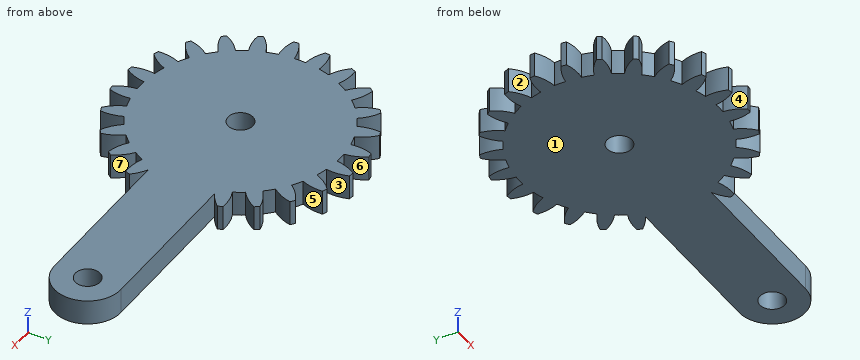
```python
from build123d import *

# Parameters (mm, degrees)
SKETCH1_R           = 1.5
BOSS_EXTRUDE1_DEPTH = 3
SCALE1_SCALE        = 1.9


with BuildPart() as part:
    # Sketch1 → Boss-Extrude1 (new body)
    with BuildSketch(Plane.XY):
        with BuildLine():
            ThreePointArc((31, -4), (35, 0), (31, 4))
            Line((31, 4), (11.967993881, 4))
            ThreePointArc((11.967993881, 4), (12.864888434, 4.573115684), (13.63194632, 5.311020574))
            ThreePointArc((13.63194632, 5.311020574), (13.516357561, 5.598658616), (13.394700346, 5.883783021))
            ThreePointArc((13.394700346, 5.883783021), (12.067442445, 5.825370588), (10.794615193, 5.444665539))
            ThreePointArc((10.794615193, 5.444665539), (10.470247132, 6.045), (10.112526268, 6.626078212))
            ThreePointArc((10.112526268, 6.626078212), (11.078640138, 7.538026423), (11.79285574, 8.658259265))
            ThreePointArc((11.79285574, 8.658259265), (11.606759368, 8.906179706), (11.415451897, 9.150101529))
            ThreePointArc((11.415451897, 9.150101529), (10.148537462, 8.750159829), (9.017614465, 8.052995056))
            ThreePointArc((9.017614465, 8.052995056), (8.548920985, 8.548920985), (8.052995056, 9.017614465))
            ThreePointArc((8.052995056, 9.017614465), (8.750159829, 10.148537462), (9.150101529, 11.415451897))
            ThreePointArc((9.150101529, 11.415451897), (8.906179706, 11.606759368), (8.658259265, 11.79285574))
            ThreePointArc((8.658259265, 11.79285574), (7.538026423, 11.078640138), (6.626078212, 10.112526268))
            ThreePointArc((6.626078212, 10.112526268), (6.045, 10.470247132), (5.444665539, 10.794615193))
            ThreePointArc((5.444665539, 10.794615193), (5.825370588, 12.067442445), (5.883783021, 13.394700346))
            ThreePointArc((5.883783021, 13.394700346), (5.598658616, 13.516357561), (5.311020574, 13.63194632))
            ThreePointArc((5.311020574, 13.63194632), (4.413811339, 12.65212943), (3.78298568, 11.482905527))
            ThreePointArc((3.78298568, 11.482905527), (3.129122255, 11.67804324), (2.465291063, 11.835980736))
            ThreePointArc((2.465291063, 11.835980736), (2.503591968, 13.163971168), (2.216494423, 14.461122103))
            ThreePointArc((2.216494423, 14.461122103), (1.909598192, 14.504838322), (1.601844607, 14.542042286))
            ThreePointArc((1.601844607, 14.542042286), (0.988802307, 13.36339701), (0.682088925, 12.070743751))
            ThreePointArc((0.682088925, 12.070743751), (0, 12.09), (-0.682088925, 12.070743751))
            ThreePointArc((-0.682088925, 12.070743751), (-0.988802307, 13.36339701), (-1.601844607, 14.542042286))
            ThreePointArc((-1.601844607, 14.542042286), (-1.909598192, 14.504838322), (-2.216494423, 14.461122103))
            ThreePointArc((-2.216494423, 14.461122103), (-2.503591968, 13.163971168), (-2.465291063, 11.835980736))
            ThreePointArc((-2.465291063, 11.835980736), (-3.129122255, 11.67804324), (-3.78298568, 11.482905527))
            ThreePointArc((-3.78298568, 11.482905527), (-4.413811339, 12.65212943), (-5.311020574, 13.63194632))
            ThreePointArc((-5.311020574, 13.63194632), (-5.598658616, 13.516357561), (-5.883783021, 13.394700346))
            ThreePointArc((-5.883783021, 13.394700346), (-5.825370588, 12.067442445), (-5.444665539, 10.794615193))
            ThreePointArc((-5.444665539, 10.794615193), (-6.045, 10.470247132), (-6.626078212, 10.112526268))
            ThreePointArc((-6.626078212, 10.112526268), (-7.538026423, 11.078640138), (-8.658259265, 11.79285574))
            ThreePointArc((-8.658259265, 11.79285574), (-8.906179706, 11.606759368), (-9.150101529, 11.415451897))
            ThreePointArc((-9.150101529, 11.415451897), (-8.750159829, 10.148537462), (-8.052995056, 9.017614465))
            ThreePointArc((-8.052995056, 9.017614465), (-8.548920985, 8.548920985), (-9.017614465, 8.052995056))
            ThreePointArc((-9.017614465, 8.052995056), (-10.148537462, 8.750159829), (-11.415451897, 9.150101529))
            ThreePointArc((-11.415451897, 9.150101529), (-11.606759368, 8.906179706), (-11.79285574, 8.658259265))
            ThreePointArc((-11.79285574, 8.658259265), (-11.078640138, 7.538026423), (-10.112526268, 6.626078212))
            ThreePointArc((-10.112526268, 6.626078212), (-10.470247132, 6.045), (-10.794615193, 5.444665539))
            ThreePointArc((-10.794615193, 5.444665539), (-12.067442445, 5.825370588), (-13.394700346, 5.883783021))
            ThreePointArc((-13.394700346, 5.883783021), (-13.516357561, 5.598658616), (-13.63194632, 5.311020574))
            ThreePointArc((-13.63194632, 5.311020574), (-12.65212943, 4.413811339), (-11.482905527, 3.78298568))
            ThreePointArc((-11.482905527, 3.78298568), (-11.67804324, 3.129122255), (-11.835980736, 2.465291063))
            ThreePointArc((-11.835980736, 2.465291063), (-13.163971168, 2.503591968), (-14.461122103, 2.216494423))
            ThreePointArc((-14.461122103, 2.216494423), (-14.504838322, 1.909598192), (-14.542042286, 1.601844607))
            ThreePointArc((-14.542042286, 1.601844607), (-13.36339701, 0.988802307), (-12.070743751, 0.682088925))
            ThreePointArc((-12.070743751, 0.682088925), (-12.09, 0), (-12.070743751, -0.682088925))
            ThreePointArc((-12.070743751, -0.682088925), (-13.36339701, -0.988802307), (-14.542042286, -1.601844607))
            ThreePointArc((-14.542042286, -1.601844607), (-14.504838322, -1.909598192), (-14.461122103, -2.216494423))
            ThreePointArc((-14.461122103, -2.216494423), (-13.163971168, -2.503591968), (-11.835980736, -2.465291063))
            ThreePointArc((-11.835980736, -2.465291063), (-11.67804324, -3.129122255), (-11.482905527, -3.78298568))
            ThreePointArc((-11.482905527, -3.78298568), (-12.65212943, -4.413811339), (-13.63194632, -5.311020574))
            ThreePointArc((-13.63194632, -5.311020574), (-13.516357561, -5.598658616), (-13.394700346, -5.883783021))
            ThreePointArc((-13.394700346, -5.883783021), (-12.067442445, -5.825370588), (-10.794615193, -5.444665539))
            ThreePointArc((-10.794615193, -5.444665539), (-10.470247132, -6.045), (-10.112526268, -6.626078212))
            ThreePointArc((-10.112526268, -6.626078212), (-11.078640138, -7.538026423), (-11.79285574, -8.658259265))
            ThreePointArc((-11.79285574, -8.658259265), (-11.606759368, -8.906179706), (-11.415451897, -9.150101529))
            ThreePointArc((-11.415451897, -9.150101529), (-10.148537462, -8.750159829), (-9.017614465, -8.052995056))
            ThreePointArc((-9.017614465, -8.052995056), (-8.548920985, -8.548920985), (-8.052995056, -9.017614465))
            ThreePointArc((-8.052995056, -9.017614465), (-8.750159829, -10.148537462), (-9.150101529, -11.415451897))
            ThreePointArc((-9.150101529, -11.415451897), (-8.906179706, -11.606759368), (-8.658259265, -11.79285574))
            ThreePointArc((-8.658259265, -11.79285574), (-7.538026423, -11.078640138), (-6.626078212, -10.112526268))
            ThreePointArc((-6.626078212, -10.112526268), (-6.045, -10.470247132), (-5.444665539, -10.794615193))
            ThreePointArc((-5.444665539, -10.794615193), (-5.825370588, -12.067442445), (-5.883783021, -13.394700346))
            ThreePointArc((-5.883783021, -13.394700346), (-5.598658616, -13.516357561), (-5.311020574, -13.63194632))
            ThreePointArc((-5.311020574, -13.63194632), (-4.413811339, -12.65212943), (-3.78298568, -11.482905527))
            ThreePointArc((-3.78298568, -11.482905527), (-3.129122255, -11.67804324), (-2.465291063, -11.835980736))
            ThreePointArc((-2.465291063, -11.835980736), (-2.503591968, -13.163971168), (-2.216494423, -14.461122103))
            ThreePointArc((-2.216494423, -14.461122103), (-1.909598192, -14.504838322), (-1.601844607, -14.542042286))
            ThreePointArc((-1.601844607, -14.542042286), (-0.988802307, -13.36339701), (-0.682088925, -12.070743751))
            ThreePointArc((-0.682088925, -12.070743751), (0, -12.09), (0.682088925, -12.070743751))
            ThreePointArc((0.682088925, -12.070743751), (0.988802307, -13.36339701), (1.601844607, -14.542042286))
            ThreePointArc((1.601844607, -14.542042286), (1.909598192, -14.504838322), (2.216494423, -14.461122103))
            ThreePointArc((2.216494423, -14.461122103), (2.503591968, -13.163971168), (2.465291063, -11.835980736))
            ThreePointArc((2.465291063, -11.835980736), (3.129122255, -11.67804324), (3.78298568, -11.482905527))
            ThreePointArc((3.78298568, -11.482905527), (4.413811339, -12.65212943), (5.311020574, -13.63194632))
            ThreePointArc((5.311020574, -13.63194632), (5.598658616, -13.516357561), (5.883783021, -13.394700346))
            ThreePointArc((5.883783021, -13.394700346), (5.825370588, -12.067442445), (5.444665539, -10.794615193))
            ThreePointArc((5.444665539, -10.794615193), (6.045, -10.470247132), (6.626078212, -10.112526268))
            ThreePointArc((6.626078212, -10.112526268), (7.538026423, -11.078640138), (8.658259265, -11.79285574))
            ThreePointArc((8.658259265, -11.79285574), (8.906179706, -11.606759368), (9.150101529, -11.415451897))
            ThreePointArc((9.150101529, -11.415451897), (8.750159829, -10.148537462), (8.052995056, -9.017614465))
            ThreePointArc((8.052995056, -9.017614465), (8.548920985, -8.548920985), (9.017614465, -8.052995056))
            ThreePointArc((9.017614465, -8.052995056), (10.148537462, -8.750159829), (11.415451897, -9.150101529))
            ThreePointArc((11.415451897, -9.150101529), (11.606759368, -8.906179706), (11.79285574, -8.658259265))
            ThreePointArc((11.79285574, -8.658259265), (11.078640138, -7.538026423), (10.112526268, -6.626078212))
            ThreePointArc((10.112526268, -6.626078212), (10.470247132, -6.045), (10.794615193, -5.444665539))
            ThreePointArc((10.794615193, -5.444665539), (12.067442445, -5.825370588), (13.394700346, -5.883783021))
            ThreePointArc((13.394700346, -5.883783021), (13.516357561, -5.598658616), (13.63194632, -5.311020574))
            ThreePointArc((13.63194632, -5.311020574), (12.864888434, -4.573115684), (11.967993881, -4))
            Line((11.967993881, -4), (31, -4))
        make_face()
        Circle(SKETCH1_R, mode=Mode.SUBTRACT)
        with Locations((31, 0)):
            Circle(SKETCH1_R, mode=Mode.SUBTRACT)
    extrude(amount=-BOSS_EXTRUDE1_DEPTH)


with BuildPart() as part_1:
    # Scale1: scaled about (5.383637445, 0, -1.5)
    add(part.part.scale(SCALE1_SCALE).moved(Location((-4.8452737, 0, 1.35))))


solid = part_1.part
```
Check sheet for the modelled part. Datum: model origin and axes. Units: mm. Face numbers are marked on the shaded views. A direction names the side the tool comes from. Round coordinates to 2 decimals unless told otherwise and drop trailing zeros. Loops run counter-clockwise (first coordinate to the right, second up) from the corner with the lowest first, then second, coordinate; pieces in that order, holes last. Notation, with made-up numbers: (84.25, 4.5) - (137.25, 4.5) arc R14 cw to (137.25, 15.5) - close; hole circle Ø9 at (51, 57). An arc over 180 degrees is marked (long way). Write item = value, one per line. Start each with the question number.
Q1. Section check C-C (z = 0.2). Count the separate pieces of the cut face and the enclosed holes in it, plus the area to 3 significant figures.
Q2. Section check D-D (x = 9). Record the boundary of the cut face in (y, z).
Q3. Release check for a two-part mould opening along Y. For the marked faces 4, 5, 6 and 7 record: pulls with the +Y half, pulls with the -Y half, needs draft (parallel to the pull), parting line crosses it, or undercut.
Q4. Access from +Z, -Z, +X, -X, +Y, -Y to the whole of each face (thin tool, end or side, straight path). Record for the marked faces 1, 2 and 3.
Q5. Section check A-A (y = 0). Record the boundary of the cut face in (x, z), plus the area to 3 significant figures.
Q6. Depth check by flat-ended pin: P1, Ø5, axis at x = -4.85, y = 0, coming from the +Z side. Enter the tip coordinate at first touch or a pass-through.
Q7. Thickness scan on L1, parallel to Y at x = -26.5, z = -2.6; L2, parallel to Y at x = -27.5, z = -2.9; L3, parallel to Y at x = -12, z = -0.35. Record the ranges inside material, lowest first.
Q8. Section check B-B (x = 47). Record the boundary of the cut face in (y, z), plus the area to 3 significant figures.
Derived:
q1.separate_pieces = 1
q1.enclosed_holes = 2
q1.area = 2,540 mm^2
q2.outline = (-20.63, -4.35) - (20.63, -4.35) - (20.63, 1.35) - (-20.63, 1.35) - close
q3.face_4 = pulls with the -Y half
q3.face_5 = undercut
q3.face_6 = pulls with the +Y half
q3.face_7 = undercut
q4.face_1 = -Z, +X, -X, +Y, -Y
q4.face_2 = +Z, -Z, -X
q4.face_3 = +Z, -Z
q5.outline = (-27.82, -4.35) - (-7.7, -4.35) - (-7.7, 1.35) - (-27.82, 1.35) - close; (-2, -4.35) - (51.2, -4.35) - (51.2, 1.35) - (-2, 1.35) - close; (56.9, -4.35) - (61.65, -4.35) - (61.65, 1.35) - (56.9, 1.35) - close
q5.area = 445 mm^2
q6.P1 = through
q7.L1 = -17.38 to -15.13, -10.77 to 10.77, 15.13 to 17.38
q7.L2 = -11.02 to -7.56, -4.71 to 4.71, 7.56 to 11.02
q7.L3 = -21.83 to 21.83
q8.outline = (-7.6, -4.35) - (7.6, -4.35) - (7.6, 1.35) - (-7.6, 1.35) - close
q8.area = 86.6 mm^2
